Source: CAD feature listing. Evaluate the final solid. Frame: model axes, mm. A direction names the side the tool comes from. Give positions to 0.01 mm unless a question says otherwise; leave off trailing zeros. Order: outer loops, then holes, each group sorted by start corner. A loop starts at its lowest first (then second) coordinate and runs counter-clockwise, first axis right, second up.
from build123d import *

# Parameters (mm, degrees)
F0_R     = 3
F1_DEPTH = 7
F3_DEPTH = 25
F5_DEPTH = 2.5


with BuildPart() as f1:
    # F0 (on Top) → F1 (new body)
    with BuildSketch(Plane.XY):
        with BuildLine():
            Line((27.09576, 2.867882), (4.09576, 2.867882))
            ThreePointArc((4.09576, 2.867882), (-5, 0), (4.09576, -2.867882))
            Line((4.09576, -2.867882), (27.09576, -2.867882))
            ThreePointArc((27.09576, -2.867882), (28.509974, -2.282096), (29.09576, -0.867882))
            Line((29.09576, -0.867882), (29.09576, 0.867882))
            ThreePointArc((29.09576, 0.867882), (28.509974, 2.282096), (27.09576, 2.867882))
        make_face()
        Circle(F0_R, mode=Mode.SUBTRACT)
    extrude(amount=F1_DEPTH)

    # F2 (on face) → F3 (cut)
    with BuildSketch(Plane.XZ.offset(2.867882)):
        with BuildLine():
            Line((23.09576, 6), (6.09576, 6))
            Line((6.09576, 6), (6.09576, 3))
            ThreePointArc((6.09576, 3), (6.681547, 1.585786), (8.09576, 1))
            Line((8.09576, 1), (25.09576, 1))
            Line((25.09576, 1), (25.09576, 4))
            ThreePointArc((25.09576, 4), (24.509974, 5.414214), (23.09576, 6))
        make_face()
    extrude(amount=-F3_DEPTH, mode=Mode.SUBTRACT)

    # F4 (on face) → F5 (cut)
    with BuildSketch(Plane.XY.offset(7)):
        with BuildLine():
            Line((-1.25, 4.841229), (-1.25, 2.727178))
            ThreePointArc((-1.25, 2.727178), (0, 3), (1.25, 2.727178))
            Line((1.25, 2.727178), (1.25, 4.841229))
            ThreePointArc((1.25, 4.841229), (0, 5), (-1.25, 4.841229))
        make_face()
        with BuildLine():
            ThreePointArc((1.25, -2.727178), (0, -3), (-1.25, -2.727178))
            Line((-1.25, -2.727178), (-1.25, -4.841229))
            ThreePointArc((-1.25, -4.841229), (0, -5), (1.25, -4.841229))
            Line((1.25, -4.841229), (1.25, -2.727178))
        make_face()
    extrude(amount=-F5_DEPTH, mode=Mode.SUBTRACT)


solid = f1.part
1) Section query B-B on y = 0. Output: boundary loops of the cut face in (x, z).
Checks:
outline: (-5, 0) - (-3, 0) - (-3, 7) - (-5, 7) - close; (3, 0) - (29.1, 0) - (29.1, 7) - (3, 7) - close; hole (6.1, 3) arc R2 ccw to (8.1, 1) - (25.1, 1) - (25.1, 4) arc R2 ccw to (23.1, 6) - (6.1, 6) - close
2) Section query A-A on x = 0. Output: boundary loops of the cut face in (y, z), and give its area (3 significant figures).
Checks:
outline: (-5, 0) - (-3, 0) - (-3, 4.5) - (-5, 4.5) - close; (3, 0) - (5, 0) - (5, 4.5) - (3, 4.5) - close
area: 18.0 mm2
3) Pull-direction query (X, two-part tool) for faces 1 (the face through (-5, 0, 3)), 2 (the face through (-3.2, 0.1, 7)), 3 (the face through (0, 4, 4.5)), 4 (the face through (29.096, 0, 3)); classes: +X half, -X half, draft (parallel to the pull), parting line (faces both ways), or undercut.
Checks:
face 1: parting line
face 2: draft
face 3: undercut
face 4: +X half
4) Reachability of faces 5 (the face through (15.8, 2.868, 6.6)), 6 (the face through (15.4, -2.868, 6.6)), 7 (the face through (1.25, 4, 6)), 8 (the face through (6.67, -0.04, 1.6)) from +Z, -Z, +X, -X, +Y, -Y: full face, straight path, thin tool, end or side. Return the list, or none.
Checks:
face 5: +Z, -Z, +X, +Y
face 6: +Z, -Z, +X, -Y
face 7: +Z, +Y, -Y
face 8: +Y, -Y
5) Ray query, L1, parallel to Y at x = 0, z = 2.75; L2, parallel to Z at x = 10.5, y = 0; L3, parallel to X at y = 0.5, z = 5. Return the intervals inside material, ascending.
Checks:
L1: y = -5 to -3, 3 to 5
L2: z = 0 to 1, 6 to 7
L3: x = -4.97 to -2.96, 2.96 to 6.1, 24.83 to 29.1
6) Section query D-D on x = 14.5. Output: boundary loops of the cut face in (y, z), and give its area (3 significant figures).
Checks:
outline: (-2.87, 0) - (2.87, 0) - (2.87, 1) - (-2.87, 1) - close; (-2.87, 6) - (2.87, 6) - (2.87, 7) - (-2.87, 7) - close
area: 11.5 mm2
7) First-contact query: pin 1 Ø0.7 at (x, y) = (0, 4) entering from +Z; pin 2 Ø2.5 at (y, z) = (-3.5, 5.5) entering from +X; pin 3 Ø1.1 at (y, z) = (-3.5, 5.5) entering from -X; pin 4 Ø3.5 at (x, y) = (0, 0) entering from +Z. Flat tips, straight axial feed; report the tip coordinate or a pass-through.
Checks:
pin 1: stops at z = 4.5
pin 2: stops at x = 28.54
pin 3: stops at x = -4.04
pin 4: passes through
8) Section query C-C on z = 2.5. Output: boundary loops of the cut face in (x, y), and give its area (3 significant figures).
Checks:
outline: (4.1, -2.87) - (6.16, -2.87) - (6.16, 2.87) - (4.1, 2.87) arc R5 ccw (long way) to start; (25.1, -2.87) - (27.1, -2.87) arc R2 ccw to (29.1, -0.87) - (29.1, 0.87) arc R2 ccw to (27.1, 2.87) - (25.1, 2.87) - close; hole circle Ø6 at (0, 0)
area: 79.8 mm2
